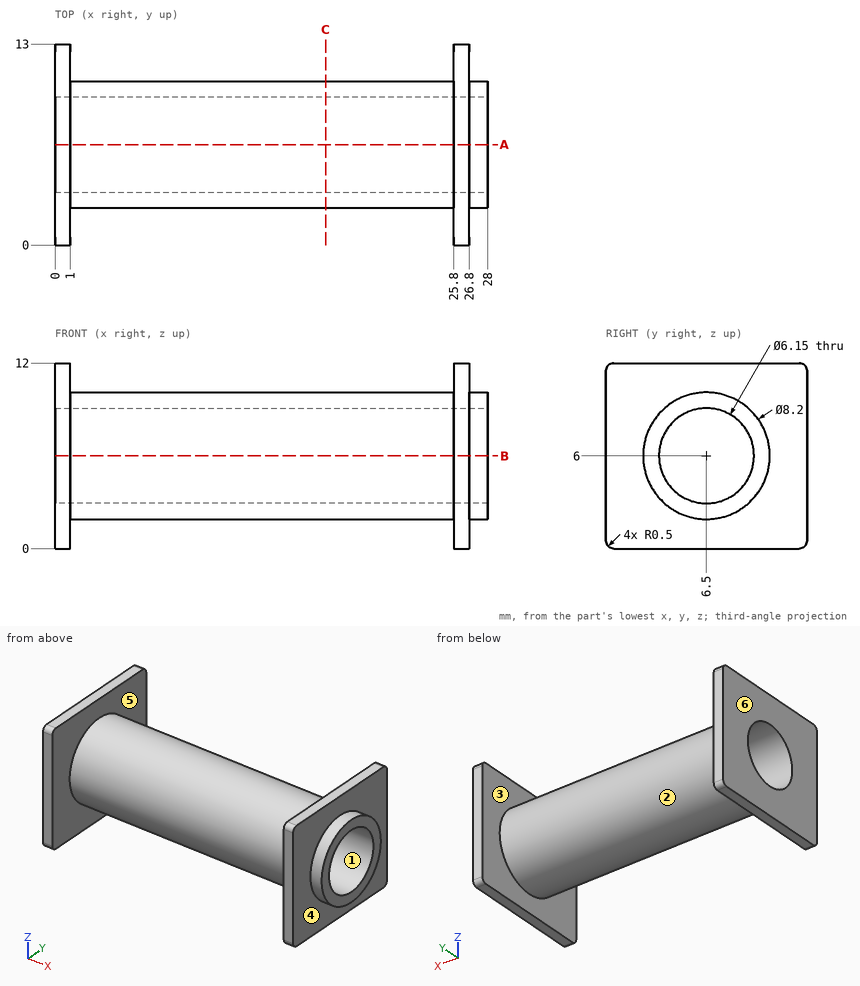
Verification items for this drawing (mm, ordinates from the low corner). A direction names the side the tool comes from. Coordinates: 2 decimals unless noted, no trailing zeros. Order: outer loops, then holes, each group sorted by start corner. A loop starts at its lowest first (then second) coordinate and runs counter-clockwise, first axis right, second up. Notation, with made-up numbers: (-32, 20.25) - (26, 20.25) arc R35 cw to (26, 53.25) - close; hole circle Ø11 at (-7, 40). An arc over 180 degrees is marked (long way). Answer in a Markdown table with one row per item. Add a question column.
1. Draft check along Y on the marked faces 1, 2 and 3. Enter one of: +Y half, -Y half, draft (parallel to the pull), parting line (faces both ways), or undercut.
2. Material ranges on L1, parallel to X at y = 9.5, z = 10; L2, parallel to Y at x = 20.75, z = 3.75; L3, parallel to Y at x = 8, z = 5, recorded low to high. Write a range as [from, to].
3. Gauge pin test, flat ends, axial feed: pin 1 Ø2 at (x, y) = (13.5, 7) entering from -Z; pin 2 Ø3.5 at (y, z) = (4, 6) entering from -X; pin 3 Ø1.5 at (x, y) = (8, 3) entering from +Z; pin 4 Ø1 at (x, y) = (11, 9.5) entering from -Z. Record the tip position at first contact, or that the pin passes through.
4. Section check B-B (z = 6). Enter the section's corners in (x, y) (3 decimals).
5. Section check A-A (y = 6.5). Enter the section's corners in (x, z) (3 decimals), plus the area to 3 significant figures.
6. Access from +Z, -Z, +X, -X, +Y, -Y to the whole of each face (thin tool, end or side, straight path). Record for the marked faces 4, 5 and 6.
7. Section check C-C (x = 17.5). Enter the section's corners in (y, z) (3 decimals).
Data:
| question | item | result |
|---|---|---|
| 1 | face 1 | undercut |
| 1 | face 2 | parting line |
| 1 | face 3 | draft |
| 2 | L1 | x = [0, 1], [25.8, 26.8] |
| 2 | L2 | y = [3.07, 4.4], [8.6, 9.93] |
| 2 | L3 | y = [2.52, 3.59], [9.41, 10.48] |
| 3 | pin 1 | stops at z = 1.9 |
| 3 | pin 2 | stops at x = 0 |
| 3 | pin 3 | stops at z = 9.04 |
| 3 | pin 4 | stops at z = 2.75 |
| 4 | outline | (0, 0) - (1, 0) - (1, 2.4) - (25.8, 2.4) - (25.8, 0) - (26.8, 0) - (26.8, 2.4) - (28, 2.4) - (28, 3.425) - (0, 3.425) - close; (0, 9.575) - (28, 9.575) - (28, 10.6) - (26.8, 10.6) - (26.8, 13) - (25.8, 13) - (25.8, 10.6) - (1, 10.6) - (1, 13) - (0, 13) - close |
| 5 | outline | (0, 0) - (1, 0) - (1, 1.9) - (25.8, 1.9) - (25.8, 0) - (26.8, 0) - (26.8, 1.9) - (28, 1.9) - (28, 2.925) - (0, 2.925) - close; (0, 9.075) - (28, 9.075) - (28, 10.1) - (26.8, 10.1) - (26.8, 12) - (25.8, 12) - (25.8, 10.1) - (1, 10.1) - (1, 12) - (0, 12) - close |
| 5 | area | 65.0 mm² |
| 6 | face 4 | +X |
| 6 | face 5 | none |
| 6 | face 6 | +Z, -Z, -X, +Y, -Y |
| 7 | outline | circle Ø8.2 at (6.5, 6); hole circle Ø6.15 at (6.5, 6) |
